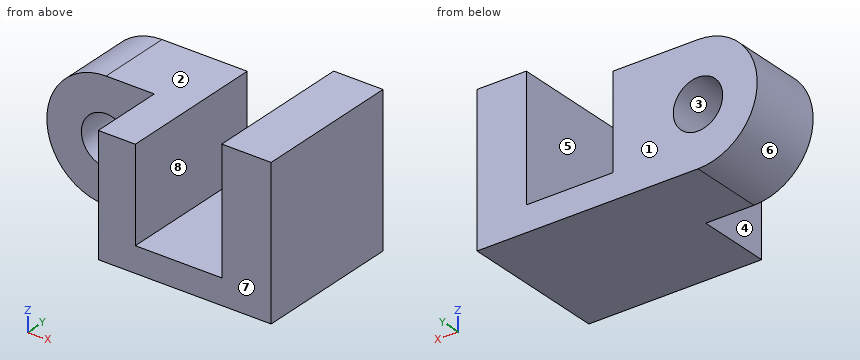
from build123d import *

# Parameters (mm, degrees)
F1_DEPTH = 600
F2_W     = 300
F2_H     = 480
F3_DEPTH = 195
F5_DEPTH = 300
F6_R     = 100
F7_DEPTH = 300.001


with BuildPart() as f1:
    # F0 (on Front) → F1 (new body)
    with BuildSketch(Plane.XZ):
        Polygon((-350, 180), (-350, -300), (350, -300), (350, 300), (150, 300), (150, -196.909353), (-200, -196.909353), (-200, 180), align=None)
    extrude(amount=F1_DEPTH)

    # F2 (on face) → F3 (join)
    with BuildSketch(Plane(origin=(-350, 0, 0), x_dir=(0, -1, 0), z_dir=(-1, 0, 0))):
        with Locations((150, -60)):
            Rectangle(F2_W, F2_H)
    extrude(amount=F3_DEPTH)

    # F4 (on face) → F5 (join)
    with BuildSketch(Plane.XZ.offset(300)):
        with BuildLine():
            ThreePointArc((-545, -300), (-375.294373, -229.705627), (-305, -60))
            ThreePointArc((-305, -60), (-375.294373, 109.705627), (-545, 180))
            Line((-545, 180), (-545, -300))
        make_face()
        with BuildLine():
            Line((-545, -300), (-545, 180))
            ThreePointArc((-545, 180), (-785, -60), (-545, -300))
        make_face()
    extrude(amount=-F5_DEPTH)

    # F6 (on face) → F7 (cut, through all)
    with BuildSketch(Plane.XZ.offset(300)):
        with Locations((-545, -60)):
            Circle(F6_R)
    extrude(amount=-F7_DEPTH, mode=Mode.SUBTRACT)


solid = f1.part
Geometry check sheet. Reference: the model listing, model coordinates, mm. Face numbers are marked on the shaded views. A direction names the side the tool comes from. Give positions to 0.01 mm unless a question says otherwise; leave off trailing zeros. Write each loop counter-clockwise with the first axis right and the second up, starting at its lowest first coordinate (ties: lowest second). Pieces come first, ordered by that corner, then holes.
1) Cross-section at B-B (y = -144.5). Record the boundary of the cut face in (x, z), plus the area to 3 significant figures.
Values follow:
outline: (-545, -300) - (350, -300) - (350, 300) - (150, 300) - (150, -196.91) - (-200, -196.91) - (-200, 180) - (-545, 180) arc R240 ccw to start; hole circle Ø200 at (-545, -60)
area: 381,000 mm2
2) Thickness scan on line 1 (Z direction, x = -545, y = -64); line 2 (X direction, y = -320, z = 89); line 3 (Y direction, x = -365.5, z = 177). Record the ranges inside material, lowest first.
Values follow:
line 1: z = -300 to -160, 40 to 180
line 2: x = -350 to -200, 150 to 350
line 3: y = -300 to 0
3) Cross-section at A-A (z = -60). Record the boundary of the cut face in (x, y).
Values follow:
outline: (-785, -300) - (-645, -300) - (-645, 0) - (-785, 0) - close; (-445, -300) - (-350, -300) - (-350, -600) - (-200, -600) - (-200, 0) - (-445, 0) - close; (150, -600) - (350, -600) - (350, 0) - (150, 0) - close
4) Cross-section at D-D (x = -568). Record the boundary of the cut face in (y, z).
Values follow:
outline: (-300, -298.9) - (0, -298.9) - (0, -157.32) - (-300, -157.32) - close; (-300, 37.32) - (0, 37.32) - (0, 178.9) - (-300, 178.9) - close
5) Release check for a two-part mould opening along X. For the marked faces 6, 7 and 8 record: released by +X, released by -X, zero draft, split by the parting line, or undercut.
Values follow:
face 6: released by -X
face 7: zero draft
face 8: undercut
6) Set-up check for the marked faces 1, 2, 3, 4 and 5: record each of +Z, -Z, +X, -X, +Y, -Y from which the full face is reachable in a straight line by a thin tool's end or side.
Values follow:
face 1: +Z, -Z, +X, -X, +Y
face 2: +Z, -X, +Y, -Y
face 3: +Y, -Y
face 4: +Z, -Z, -X, -Y
face 5: +Z, +Y, -Y
7) Go/stop test with flat-tipped pins: pin 1 Ø8 at (x, y) = (-55.5, -474.5) entering from +Z; pin 2 Ø6 at (y, z) = (-481.5, 206) entering from -X; pin 3 Ø2 at (x, y) = (-205.5, -272.5) entering from +Z. Record where each tip stops, or that it passes through.
Values follow:
pin 1: stops at z = -196.91
pin 2: stops at x = 150
pin 3: stops at z = 180
8) Cross-section at C-C (z = 94). Record the boundary of the cut face in (x, y), plus the area to 3 significant figures.
Values follow:
outline: (-729.08, -300) - (-350, -300) - (-350, -600) - (-200, -600) - (-200, 0) - (-729.08, 0) - close; (150, -600) - (350, -600) - (350, 0) - (150, 0) - close
area: 324,000 mm2
